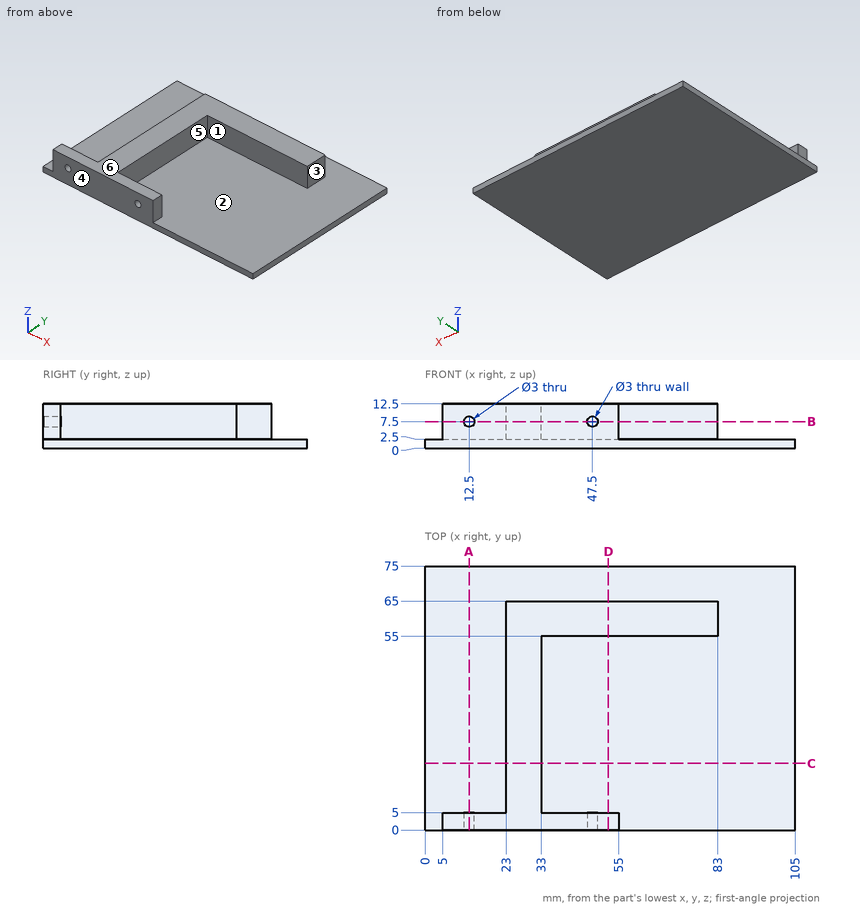
Study the drawing (mm; zero at the part's minimum x, y, z) and answer. A direction names the side the tool comes from. Give positions to 0.01 mm unless a question says otherwise; leave off trailing zeros. Write each loop counter-clockwise with the first axis right and the second up, starting at its lowest first coordinate (ties: lowest second). Pieces come first, ordered by that corner, then holes. Notation, with made-up numbers: (79.5, -29.5) - (115.5, -29.5) arc R22 cw to (115.5, -7.5) - close; hole circle Ø7 at (-28.75, 74.25). An arc over 180 degrees is marked (long way). Write item = value, one per line. Start each with the question number.
Item 1: A tool of negligible diameter and unlimited length cuts with its end or side. For the marked faces 5 and 6, from which of +Z, -Z, +X, -X, +Y, -Y can it reach the whole face along a straight path? Write none if from no direction.
Item 2: Find section C-C (y = 19). Give the vertices of the cut face in (x, z), then the cut area to 4 significant figures.
Item 3: Find the intervals of material crossed by probe 1 along Y at (x, z) = (41, 10.25); probe 2 along Z at (x, y) = (47.5, 3.4); probe 3 along Z at (x, y) = (39, 28), in increasing order. Write a range as [from, to].
Item 4: Each of these flat-tipped pins is pushed along its axis until it touches: P1, Ø5, axis at y = 27, z = 5.5, coming from the -X side; P2, Ø5, axis at x = 63, z = 7.5, coming from the -Y side; P3, Ø4, axis at x = 70.5, y = 21, coming from the +Z side. Where does it stop, or does it pass through?
Item 5: The mould has two halves that part along Y. Classify the marked faces 1, 2, 3 and 4: +Y half, -Y half, draft (parallel to the pull), parting line (faces both ways), or undercut.
Item 6: Find section D-D (x = 52). Give the vertices of the cut face in (y, z), then the cut area to 4 significant figures.
Item 7: Find section B-B (z = 7.5). Give the vertices of the cut face in (x, y), then the cut area to 3 significant figures.
Item 8: Find section A-A (x = 12.5). Give the vertices of the cut face in (y, z), then the cut area to 4 significant figures.
Response:
q1.face_5 = +Z, +X
q1.face_6 = +Z, +X, -X, +Y, -Y
q2.outline = (0, 0) - (105, 0) - (105, 2.5) - (33, 2.5) - (33, 12.5) - (23, 12.5) - (23, 2.5) - (0, 2.5) - close
q2.area = 362.5 mm²
q3.probe_1 = [0, 5], [55, 65]
q3.probe_2 = [0, 6], [9, 12.5]
q3.probe_3 = [0, 2.5]
q4.P1 = 23
q4.P2 = 55
q4.P3 = 2.5
q5.face_1 = undercut
q5.face_2 = undercut
q5.face_3 = draft
q5.face_4 = -Y half
q6.outline = (0, 0) - (75, 0) - (75, 2.5) - (65, 2.5) - (65, 12.5) - (55, 12.5) - (55, 2.5) - (5, 2.5) - (5, 12.5) - (0, 12.5) - close
q6.area = 337.5 mm²
q7.outline = (5, 0) - (11, 0) - (11, 5) - (5, 5) - close; (14, 0) - (46, 0) - (46, 5) - (33, 5) - (33, 55) - (83, 55) - (83, 65) - (23, 65) - (23, 5) - (14, 5) - close; (49, 0) - (55, 0) - (55, 5) - (49, 5) - close
q7.area = 1,320 mm²
q8.outline = (0, 0) - (75, 0) - (75, 2.5) - (5, 2.5) - (5, 6) - (0, 6) - close; (0, 9) - (5, 9) - (5, 12.5) - (0, 12.5) - close
q8.area = 222.5 mm²
